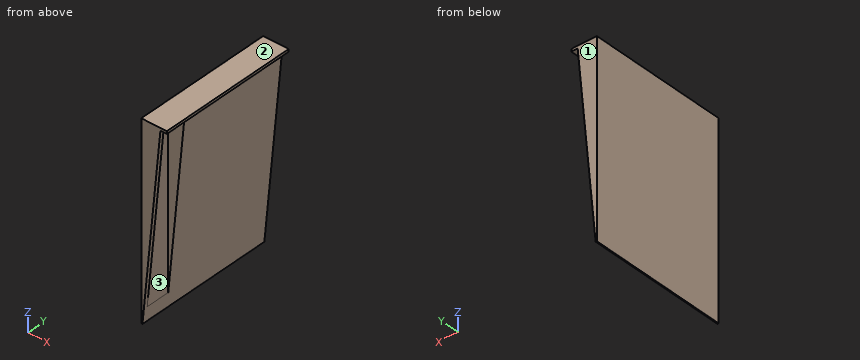
from build123d import *

# Parameters (mm, degrees)
F1_DEPTH = 110
F3_W     = 19
F3_H     = 148
F4_DEPTH = 18.001


with BuildPart() as f1:
    # F0 (on Front) → F1 (new body)
    with BuildSketch(Plane.XZ):
        Polygon((20, 17.5948), (0, 17.5948), (0, -132.4052), (0.90309, -132.4052), (15, 15.5948), (20, 15.5948), align=None)
    extrude(amount=F1_DEPTH)

    # F3 (on offset) → F4 (cut, through all)
    with BuildSketch(Plane.YZ.offset(2)):
        with Locations((-97.5, -58.4052)):
            Rectangle(F3_W, F3_H)
    extrude(amount=F4_DEPTH, mode=Mode.SUBTRACT)


solid = f1.part
The model under review builds one solid part; all positions refer to its coordinate system, in mm. Face numbers are marked on the shaded views. Coordinates: 2 decimals unless noted, no trailing zeros. Write each loop counter-clockwise with the first axis right and the second up, starting at its lowest first coordinate (ties: lowest second). Pieces come first, ordered by that corner, then holes. Notation, with made-up numbers: (-3.75, 59) -> (18.25, 59) arc R18 cw to (18.25, 80) -> close; hole circle Ø5 at (35.25, 58). An arc over 180 degrees is marked (long way). Answer in a Markdown table with one row per item.
1. We need section C-C, the plane z = -65.5. State the section outline as (x, y) points, and give its area (3 significant figures).
Answers below:
| item | result |
|---|---|
| outline | (0, -110) -> (7.28, -110) -> (7.28, -107) -> (2, -107) -> (2, -88) -> (7.28, -88) -> (7.28, 0) -> (0, 0) -> close |
| area | 700 mm^2 |
2. We need section D-D, the plane y = -62.5. State the section outline as (x, z) points, and give its area (3 significant figures).
Answers below:
| item | result |
|---|---|
| outline | (0, -132.41) -> (0.9, -132.41) -> (15, 15.59) -> (20, 15.59) -> (20, 17.59) -> (0, 17.59) -> close |
| area | 1,220 mm^2 |
3. Draft analysis for pull direction Y (two halves, no side actions). For the marked faces 1, 2 and 3, state which applies: +Y half, -Y half, draft (parallel to the pull), parting line (faces both ways), or undercut.
Answers below:
| item | result |
|---|---|
| face 1 | +Y half |
| face 2 | draft |
| face 3 | undercut |
4. Clearance check with flat-ended pins moving along their axes: pin 1 Ø12 at (y, z) = (-21.5, -48.5) entering from +X; pin 2 Ø6 at (y, z) = (-86, -113) entering from +X; pin 3 Ø12 at (x, z) = (6, -99) entering from +Y; pin 4 Ø5.5 at (y, z) = (-94, -45.5) entering from +X. State where each tip first meets the part, or that it passes through.
Answers below:
| item | result |
|---|---|
| pin 1 | stops at x = 9.47 |
| pin 2 | stops at x = 3.04 |
| pin 3 | stops at y = 0 |
| pin 4 | stops at x = 2 |
5. We need section B-B, the plane x = 4. State the section outline as (y, z) points.
Answers below:
| item | result |
|---|---|
| outline | (-110, -99.89) -> (-107, -99.89) -> (-107, 15.59) -> (-88, 15.59) -> (-88, -99.89) -> (0, -99.89) -> (0, 17.59) -> (-110, 17.59) -> close |
6. Wall thickness on probe 1 along Y at (x, z) = (4, -97.5); probe 2 along Z at (x, y) = (18.25, -9.5); probe 3 along X at (y, z) = (-49.5, -56): over which ranges is each line inside the solid? List them lowest first. Write a range as [from, to].
Answers below:
| item | result |
|---|---|
| probe 1 | y = [-110, -107], [-88, 0] |
| probe 2 | z = [15.59, 17.59] |
| probe 3 | x = [0, 8.18] |
7. We need section A-A, the plane y = -100. State the section outline as (x, z) points.
Answers below:
| item | result |
|---|---|
| outline | (0, -132.41) -> (0.9, -132.41) -> (2, -120.89) -> (2, 15.59) -> (20, 15.59) -> (20, 17.59) -> (0, 17.59) -> close |
